Input: dimensioned drawing with shaded views. Units: mm. Origin: part minimum x, y, z. Round coordinates to 2 decimals unless told otherwise and drop trailing zeros. Order: outer loops, then holes, each group sorted by start corner. A loop starts at its lowest first (then second) coordinate and runs counter-clockwise, first axis right, second up. Notation, with made-up numbers: (49, 11.25) - (65, 11.25) arc R9 ccw to (65, 21.25) - close; hole circle Ø4 at (84.5, 27.5). An arc over 180 degrees is marked (long way). Return JSON: item names as keys, results as strings. Group by question number.
1) Section B-B, the plane z = 3.1. Return loops of the section in (x, y), plus the area to 3 significant figures.
2) Section C-C, the plane x = 46. Return loops of the section in (y, z).
3) Ray query, line 1 (Y direction, x = 29.5, z = 3.2); line 2 (X direction, y = 52.5, z = 4.6); line 3 (X direction, y = 39, z = 1.25). Return the intervals inside material, ascending. Write a range as from..to.
4) Contact query for flat-ended pins moving along their axis: P1, Ø2.5, axis at y = 3, z = 3, coming from the -X side; P2, Ø0.6, axis at x = 56.5, z = 3.5, coming from the +Y side; P3, Ø2.5, axis at y = 77, z = 1.5, coming from the +X side. Output: stop coordinate, or through.
5) Section A-A, the plane y = 22. Return loops of the section in (x, z), plus the area to 3 significant figures.
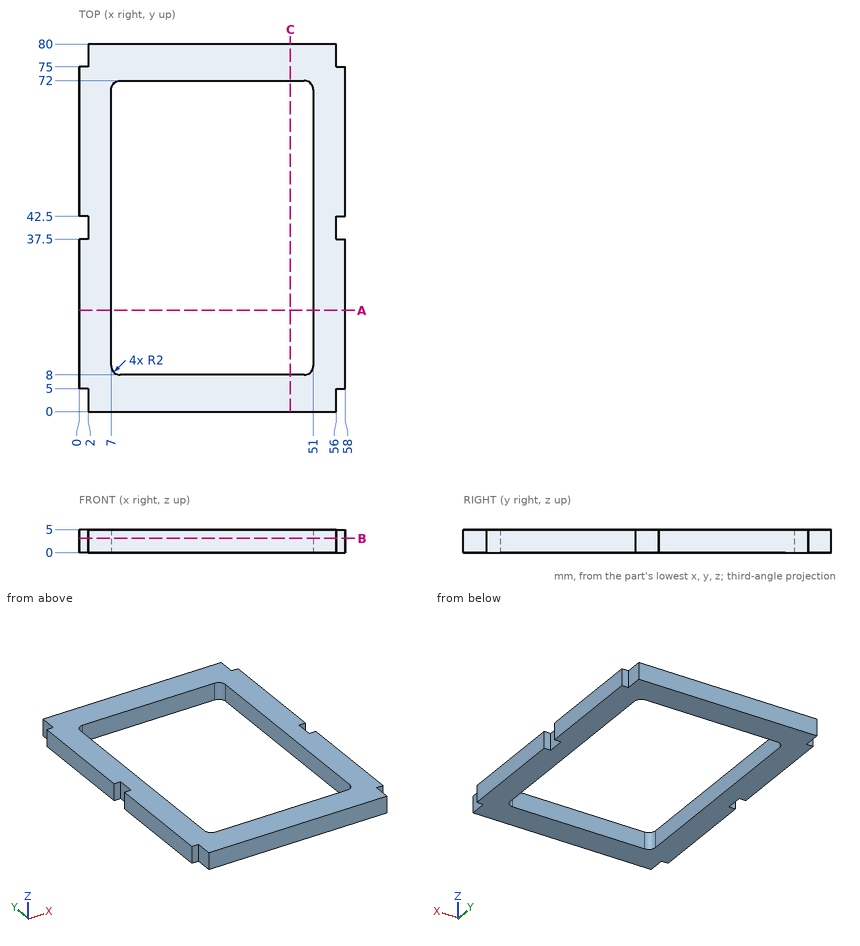
Geometry check:
{
 "1": {"outline": "(0, 5) - (2, 5) - (2, 0) - (56, 0) - (56, 5) - (58, 5) - (58, 37.5) - (56, 37.5) - (56, 42.5) - (58, 42.5) - (58, 75) - (56, 75) - (56, 80) - (2, 80) - (2, 75) - (0, 75) - (0, 42.5) - (2, 42.5) - (2, 37.5) - (0, 37.5) - close; hole (7, 10) arc R2 ccw to (9, 8) - (49, 8) arc R2 ccw to (51, 10) - (51, 70) arc R2 ccw to (49, 72) - (9, 72) arc R2 ccw to (7, 70) - close", "area": "1,770 mm2"},
 "2": {"outline": "(0, 0) - (8, 0) - (8, 5) - (0, 5) - close; (72, 0) - (80, 0) - (80, 5) - (72, 5) - close"},
 "3": {"line 1": "0..8, 72..80", "line 2": "0..7, 51..58", "line 3": "2..7, 51..56"},
 "4": {"P1": "x = 2", "P2": "y = 75", "P3": "x = 56"},
 "5": {"outline": "(0, 0) - (7, 0) - (7, 5) - (0, 5) - close; (51, 0) - (58, 0) - (58, 5) - (51, 5) - close", "area": "70.0 mm2"}
}
